Design review of the part built by this model. Coordinates are the model's own, in mm. A direction names the side the tool comes from. Coordinates: 2 decimals unless noted, no trailing zeros. Loops run counter-clockwise (first coordinate to the right, second up) from the corner with the lowest first, then second, coordinate; pieces in that order, holes last. Notation, with made-up numbers: (29.5, 39) -> (65.5, 39) arc R9 cw to (65.5, 43) -> close; hole circle Ø7 at (5.5, -27). An arc over 180 degrees is marked (long way). One line per item, written item: value. Start each with the question number.
1. Add section C-C on z = 157. Write out the cut boundary in (x, y).
2. For probe 1 along Y at (x, z) = (-271.5, 574); probe 2 along X at (y, z) = (62, 281), list the stretches that pass through material, from the lowest coordinate up.
3. Machinability: for faces 1 (the flat face through (-294, 12.7, 309)), 2 (the flat face through (-442, 6, 609.6)), which of the approach directions +Z, -Z, +X, -X, +Y, -Y give a long, thin tool a straight path to every point of the face, cutting with its end or side? Answer none if there is none.
4. Add section A-A on x = -156.5. Write out the cut boundary in (y, z), plus the area to 3 significant figures.
5. Insertion check: pin 1 (3 mm diameter, centred on x = -543, z = 201, fed in from +Y); pin 2 (10 mm diameter, centred on y = 107, z = 401, fed in from +X). Each pin has a flat end and moves straight along its axis. Give the tip position at first contact, or say it passes through.
6. Add section B-B on y = 112.5. Write out the cut boundary in (x, z).
Autodesk Inventor part; units mm, degrees
ref_plane "YZ Plane" through (0, 0, 0) normal (1, 0, 0) x (0, 1, 0)
ref_plane "XZ Plane" through (0, 0, 0) normal (0, 1, 0) x (-1, 0, 0)
ref_plane "XY Plane" through (0, 0, 0) normal (0, 0, 1) x (1, 0, 0)
sketch "Sketch1" plane through (0, 0, 0) normal (0, 1, 0) x (-1, 0, 0)
  line L0 (0, 0) -> (609.6, 0)
  line L1 (609.6, 0) -> (609.6, 609.6)
  line L2 (609.6, 609.6) -> (0, 609.6)
  line L3 (0, 609.6) -> (0, 0)
  dimension "d0" = 609.6
  dimension "d1" = 609.6
extrude "Extrusion1" add sketch "Sketch1" along normal blind 12.7
sketch "Sketch2" plane through (0, 12.7, 0) normal (0, 1, 0) x (1, 0, 0)
  line L0 (0, 0) -> (-609.6, 0)
  line L1 (-609.6, 0) -> (-596.9, 0)
  line L2 (-596.9, 0) -> (-596.9, -609.6)
  line L3 (-596.9, -609.6) -> (-609.6, -609.6)
  line L4 (-609.6, -609.6) -> (-609.6, 0)
  dimension "d4" = 12.7
  dimension "d5" = 609.6
extrude "Extrusion2" add sketch "Sketch2" along normal blind 355.6
properties part number "foam-tile"
Worked answers:
1. outline: (-609.6, 0) -> (0, 0) -> (0, 12.7) -> (-596.9, 12.7) -> (-596.9, 368.3) -> (-609.6, 368.3) -> close
2. probe 1: y = 0 to 12.7
2. probe 2: x = -609.6 to -596.9
3. face 1: +Z, -Z, +X, +Y
3. face 2: +Z, +X, -X, +Y, -Y
4. outline: (0, 0) -> (12.7, 0) -> (12.7, 609.6) -> (0, 609.6) -> close
4. area: 7,740 mm²
5. pin 1: stops at y = 12.7
5. pin 2: stops at x = -596.9
6. outline: (-609.6, 0) -> (-596.9, 0) -> (-596.9, 609.6) -> (-609.6, 609.6) -> close
